```python
from build123d import *

# Parameters (mm, degrees)
SKETCH_1_W      = 220
SKETCH_1_H      = 180
SKETCH_1_R      = 5
EXTRUDE_1_DEPTH = 10
EXTRUDE_1_DRAFT = 1
FILLET_1_R      = 5
CHAMFER_1_SIZE  = 10
CHAMFER_1_SIZE2 = 62.953374933
FILLET_2_R      = 700


with BuildPart() as part:
    # 草图1 → 凸台-拉伸1 (with draft: the straight prism first)
    with BuildSketch(Plane(origin=(0, 0, 0), x_dir=(1, 0, 0), z_dir=(0, 1, 0))):
        Rectangle(SKETCH_1_W, SKETCH_1_H)
        with Locations((-75, -61.363636364)):
            Circle(SKETCH_1_R, mode=Mode.SUBTRACT)
        with Locations((75, -61.363636364)):
            Circle(SKETCH_1_R, mode=Mode.SUBTRACT)
    extrude(amount=EXTRUDE_1_DEPTH)
    # 凸台-拉伸1: the draft: its side faces are tilted about the plane it starts from
    extrude_1_sides = [part.faces().sort_by_distance(p)[0] for p in [
        (0, 5, 90),
        (110, 5, 0),
        (0, 5, -90),
        (-110, 5, 0),
        (-80, 5, 61.363636364),
        (70, 5, 61.363636364),
    ]]
    draft(extrude_1_sides, Plane(origin=(0, 0, 0), x_dir=(1, 0, 0), z_dir=(0, 1, 0)), EXTRUDE_1_DRAFT)

    # 圆角1
    fillet_1_edges = [part.edges().sort_by_distance(p)[0] for p in [
        (109.912724675, 5, 89.912724675),
        (-109.912724675, 5, 89.912724675),
    ]]
    fillet(fillet_1_edges, radius=FILLET_1_R)

    # 倒角1
    chamfer_1_edges = [part.edges().sort_by_distance(p)[0] for p in [
        (0, 10, -89.825449351),
    ]]
    chamfer_1_side = [part.faces().sort_by_distance(p)[0] for p in [
        (0, 4.998676597, -89.912747775),
    ]]
    chamfer(chamfer_1_edges, length=CHAMFER_1_SIZE, length2=CHAMFER_1_SIZE2, reference=chamfer_1_side[0])

    # 圆角2
    fillet_2_edges = [part.edges().sort_by_distance(p)[0] for p in [
        (0, 10, -26.872074418),
    ]]
    fillet(fillet_2_edges, radius=FILLET_2_R)


solid = part.part
```
For this review, take the finished solid that the model builds, in its own axes (mm). A direction names the side the tool comes from. Coordinates: 2 decimals unless noted, no trailing zeros. Write each loop counter-clockwise with the first axis right and the second up, starting at its lowest first coordinate (ties: lowest second). Pieces come first, ordered by that corner, then holes. Notation, with made-up numbers: (19.5, 72) - (42.5, 72) arc R19 cw to (42.5, 105) - close; hole circle Ø11 at (-11, 14.5). An arc over 180 degrees is marked (long way). Answer in a Markdown table with one row per item. Add a question column.
Q1. We need section C-C, the plane z = -19. State the section outline as (x, y) points, and give its area (3 significant figures).
Q2. We need section B-B, the plane y = 3. Count the separate pieces of the cut face and the enclosed holes in it, and give its area (3 significant figures).
Q3. Draft analysis for pull direction X (two halves, no side actions). For faces 1 (the cylindrical face through (-108.486, 5.081, 88.408)), 2 (the flat face through (-1.5, 0.7, -85.6)), 3 (the conical face through (-72.7, 4.9, 65.9)), state which applies: +X half, -X half, draft (parallel to the pull), parting line (faces both ways), or undercut.
Q4. For P1, Ø3, axis at y = 3, z = 25, coming from the +X side; P2, Ø6, axis at y = 5.5, z = 44, coming from the -X side, all flat-tipped, find the tip position at first contact; note any pin that passes through.
Q5. We need section D-D, the plane z = 14. State the section outline as (x, y) points.
Q6. Tool access review of faces 4 (the conical face through (73.9, 4.93, 66.33)), 5 (the cylindrical face through (108.408, 5.081, 88.486)), 6 (the flat face through (-2, 0, -1)): name each direction out of +Z, -Z, +X, -X, +Y, -Y from which nothing blocks a thin tool from reaching the whole face with its end or side.
Q7. For probe 1 along X at (y, z) = (1.5, 75.5); probe 2 along X at (y, z) = (9, 9.5); probe 3 along Y at (x, z) = (88, -81), list the stretches that pass through material, from the lowest coordinate up.
Answer list:
| question | item | result |
|---|---|---|
| 1 | outline | (-110, 0) - (110, 0) - (109.85, 8.41) - (-109.85, 8.41) - close |
| 1 | area | 1,850 mm2 |
| 2 | separate pieces | 1 |
| 2 | enclosed holes | 2 |
| 2 | area | 35,100 mm2 |
| 3 | face 1 | -X half |
| 3 | face 2 | draft |
| 3 | face 3 | undercut |
| 4 | P1 | stops at x = 109.97 |
| 4 | P2 | stops at x = -109.96 |
| 5 | outline | (-110, 0) - (110, 0) - (109.83, 9.86) - (-109.83, 9.86) - close |
| 6 | face 4 | +Y |
| 6 | face 5 | +Z, +X, +Y |
| 6 | face 6 | +Z, -Z, +X, -X, -Y |
| 7 | probe 1 | x = -109.97 to 109.97 |
| 7 | probe 2 | x = -109.84 to 109.84 |
| 7 | probe 3 | y = 0 to 1.43 |
